Input: part model. Units: mm. Frame: model coordinates. A direction names the side the tool comes from. Give positions to 0.01 mm unless a question says otherwise; leave off trailing zeros. Loops run counter-clockwise (first coordinate to the right, second up) from the corner with the lowest first, then second, coordinate; pieces in that order, holes last. Notation, with made-up numbers: (72, 23) -> (89, 23) arc R14 ccw to (89, 43) -> close; hole circle Ø9 at (8.5, 31). An arc over 180 degrees is marked (long way). Answer as a JSON object with one key per item and string values.
Autodesk Inventor part; units mm, degrees
ref_plane "YZ Plane" through (0, 0, 0) normal (1, 0, 0) x (0, 1, 0)
ref_plane "XZ Plane" through (0, 0, 0) normal (0, 1, 0) x (-1, 0, 0)
ref_plane "XY Plane" through (0, 0, 0) normal (0, 0, 1) x (1, 0, 0)
sketch "Sketch1" plane through (0, 0, 0) normal (0, 0, 1) x (1, 0, 0)
  line L0 (-185, -300) -> (185, -300)
  line L1 (200, -285) -> (200, 285)
  line L2 (185, 300) -> (-185, 300)
  line L3 (-200, 285) -> (-200, -285)
  line L4 (-200, -300) -> (200, 300) construction
  line L5 (200, -300) -> (-200, 300) construction
  arc A0 (-185, 300) -> (-200, 285) centre (-185, 285) ccw
  arc A1 (200, 285) -> (185, 300) centre (185, 285) ccw
  arc A2 (185, -300) -> (200, -285) centre (185, -285) ccw
  arc A3 (-200, -285) -> (-185, -300) centre (-185, -285) ccw
  line L6 (-160, -235) -> (-160, 145.389)
  line L7 (-132.5192, 153.7095) -> (121.0734, -226.6795)
  line L8 (108.5926, -250) -> (-145, -250)
  line L9 (-121.0734, 226.6795) -> (132.5192, -153.7095)
  line L10 (160, -145.389) -> (160, 235)
  line L11 (145, 250) -> (-108.5926, 250)
  arc A4 (-132.5192, 153.7095) -> (-160, 145.389) centre (-145, 145.389) ccw
  arc A5 (-108.5926, 250) -> (-121.0734, 226.6795) centre (-108.5926, 235) ccw
  arc A6 (108.5926, -250) -> (121.0734, -226.6795) centre (108.5926, -235) ccw
  arc A7 (132.5192, -153.7095) -> (160, -145.389) centre (145, -145.389) ccw
  arc A8 (160, 235) -> (145, 250) centre (145, 235) ccw
  arc A9 (-160, -235) -> (-145, -250) centre (-145, -235) ccw
  circle A10 centre (-170, 270) radius 12.5
  line L12 (0, -424.3492) -> (0, 424.3492)
  line L13 (-284.3492, 0) -> (284.3492, 0)
  circle A11 centre (170, 270) radius 12.5
  circle A12 centre (-170, -270) radius 12.5
  circle A13 centre (170, -270) radius 12.5
  point P0 (0, 0)
  dimension "width" = 400
  dimension "depth" = 600
  dimension "outerCornnerRadius" = 15
  dimension "d5" = 15
  dimension "d7" = 50
  dimension "d8" = 50
  dimension "innerCorrerRadius" = 15
  dimension "d14" = 40
  dimension "d15" = 40
  dimension "d16" = 40
  dimension "d17" = 40
  dimension "d20" = 25
  dimension "d21" = 30
  dimension "d22" = 30
extrude "Extrusion3" add sketch "Sketch1" along normal blind 10 contours A3 L3 L13 L6 A9 L8 L12 L0 | L12 L8 A6 L7 L13 L9 A7 L10 L1 A2 L0 | L3 A0 L2 L12 L11 A5 L9 L13 L7 A4 L6 | L7 L13 L12 | L13 L10 A8 L11 L12 L2 A1 L1 | L12 L9 L13
equation "\"d5\" = outerCornnerRadius"
equation "\"d15\" = d14"
properties part number "pompression_plate"
Q1. Section C-C, the plane z = 1.5. Return the cut outline in (x, y).
Evaluation:
{"outline": "(-200, -285) arc R15 ccw to (-185, -300) -> (185, -300) arc R15 ccw to (200, -285) -> (200, 285) arc R15 ccw to (185, 300) -> (-185, 300) arc R15 ccw to (-200, 285) -> close; hole circle Ø25 at (-170, -270); hole circle Ø25 at (-170, 270); hole (-160, -235) arc R15 ccw to (-145, -250) -> (108.59, -250) arc R15 ccw to (121.07, -226.68) -> (-132.52, 153.71) arc R15 ccw to (-160, 145.39) -> close; hole (-121.07, 226.68) -> (132.52, -153.71) arc R15 ccw to (160, -145.39) -> (160, 235) arc R15 ccw to (145, 250) -> (-108.59, 250) arc R15 ccw to start; hole circle Ø25 at (170, -270); hole circle Ø25 at (170, 270)"}
Q2. Ray query, line 1 along Y through (x, z) = (170, 6.25); line 2 along Y through (x, z) = (73, 3); line 3 along X through (y, z) = (12, 1). Return the intervals inside material, ascending.
Evaluation:
{"line 1": "y = -300 to -282.5, -257.5 to 257.5, 282.5 to 300", "line 2": "y = -300 to -250, -154.57 to -64.43, 250 to 300", "line 3": "x = -200 to -160, -38.05 to 22.05, 160 to 200"}
Q3. Section B-B, the plane y = -270. Return the cut outline in (x, z).
Evaluation:
{"outline": "(-200, 0) -> (-182.5, 0) -> (-182.5, 10) -> (-200, 10) -> close; (-157.5, 0) -> (157.5, 0) -> (157.5, 10) -> (-157.5, 10) -> close; (182.5, 0) -> (200, 0) -> (200, 10) -> (182.5, 10) -> close"}
Q4. Access query for faces 5 (the flat face through (-3, 4, 0)), 6 (the cylindrical face through (149.603, -159.665, 4.93)). Directions: +Z, -Z, +X, -X, +Y, -Y. A direction counts if a zero-diameter tool reaches every point of the face in a straight line with its end or side. Return the directions, or none.
Evaluation:
{"face 5": "-Z, +X, -X, +Y, -Y", "face 6": "+Z, -Z"}
Q5. Pin query (flat end, axial travel): pin 1 (6 mm diameter, centred on x = -158, y = 106, fed in from -Z). Return the tip coordinate at first contact, or that it passes through.
Evaluation:
{"pin 1": "stops at z = 0"}
Q6. Draft query along X for faces 1 (the cylindrical face through (121.92, -241.88, 4.93)), 2 (the cylindrical face through (181.923, -273.755, 4.93)), 3 (the cylindrical face through (-195.72, 295.49, 4.93)), 4 (the flat face through (-3, 4, 10)). Return one class per face: +X half, -X half, draft (parallel to the pull), parting line (faces both ways), or undercut.
Evaluation:
{"face 1": "undercut", "face 2": "undercut", "face 3": "-X half", "face 4": "draft"}
Q7. Section A-A, the plane x = -170. Return the cut outline in (y, z).
Evaluation:
{"outline": "(-300, 0) -> (-282.5, 0) -> (-282.5, 10) -> (-300, 10) -> close; (-257.5, 0) -> (257.5, 0) -> (257.5, 10) -> (-257.5, 10) -> close; (282.5, 0) -> (300, 0) -> (300, 10) -> (282.5, 10) -> close"}
